Check sheet for the modelled part. Datum: model origin and axes. Units: mm. Face numbers are marked on the shaded views. Round coordinates to 2 decimals unless told otherwise and drop trailing zeros. Order: outer loops, then holes, each group sorted by start corner. A loop starts at its lowest first (then second) coordinate and runs counter-clockwise, first axis right, second up.
Q1. Cross-section at D-D on y = 11. Give the number of separate pieces and of enclosed holes in the cut face, then the cut area to 3 significant figures.
Q2. Cross-section at A-A on x = -100. Record the cut outline in (y, z).
Q3. Cross-section at B-B on z = 20.5. Record the cut outline in (x, y).
Q4. Depth check by flat-ended pin: P1, Ø1.8, axis at x = 0, z = 10, coming from the -Y side; P2, Ø5.5, axis at x = 0, z = -44, coming from the +Y side; P3, Ø3, axis at x = -90.5, y = 10, coming from the -Z side; P4, Ø5, axis at y = 2.5, z = -14.5, coming from the +X side. Enter the tip coordinate at first touch or a pass-through.
Q5. Scan lines: probe 1 along Z at (x, y) = (-70, 9.25); probe 2 along Z at (x, y) = (-70.5, 11.75); probe 3 along X at (y, z) = (7.25, -6). Record each from-to range of solid material in increasing order.
Q6. Cross-section at C-C on x = -53.5. Record the cut outline in (y, z).
Q7. Mould release check, pull along X, two halves, no side actions. Record for the marked faces 1, 2 and 3: +X half, -X half, draft (parallel to the pull), parting line (faces both ways), or undercut.
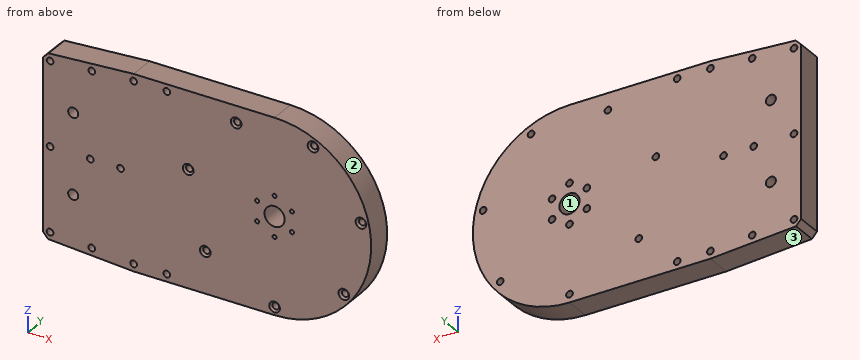
from build123d import *
from OCP.BRepFilletAPI import BRepFilletAPI_MakeChamfer

# Parameters (mm, degrees)
SKETCH1_R                 = 5
SKETCH1_R_2               = 1
BOSS_EXTRUDE1_DEPTH       = 12.7
SKETCH3_R                 = 1
CUT_EXTRUDE1_DEPTH        = 6.35
M4X0_7_TAPPED_HOLE1_D     = 3.3
CHAMFER1_SIZE             = 1
M4X0_7_TAPPED_HOLE2_D     = 3.3
M4X0_7_TAPPED_HOLE2_DEPTH = 10.1
M4X0_7_TAPPED_HOLE2_TIP   = 0.991420021
CHAMFER2_SIZE             = 2.5
CHAMFER2_SIZE2            = 2.68451721
SKETCH7_R                 = 0.25
SKETCH7_R_2               = 1
CUT_EXTRUDE2_DEPTH        = 126.26088775
M4X0_7_TAPPED_HOLE3_D     = 3.3
M4X0_7_TAPPED_HOLE3_DEPTH = 15.5
M4X0_7_TAPPED_HOLE3_TIP   = 0.991420021
M6X1_0_TAPPED_HOLE1_D     = 5
M6X1_0_TAPPED_HOLE1_DEPTH = 17
M6X1_0_TAPPED_HOLE1_TIP   = 1.502151548


with BuildPart() as part:
    # Sketch1 → Boss-Extrude1 (new body)
    with BuildSketch(Plane(origin=(0, 0, 0), x_dir=(1, 0, 0), z_dir=(0, 1, 0))):
        with BuildLine():
            Line((-115, 45), (-115, -45))
            Line((-115, -45), (-70, -48))
            Line((-70, -48), (0, -48))
            ThreePointArc((0, -48), (48, 0), (0, 48))
            Line((0, 48), (-70, 48))
            Line((-70, 48), (-115, 45))
        make_face()
        with Locations(Location((0, 0, 0), (0, 0, 270))):
            Circle(SKETCH1_R, mode=Mode.SUBTRACT)
        with Locations(Location((0, 10, 0), (0, 0, 270))):
            Circle(SKETCH1_R_2, mode=Mode.SUBTRACT)
        with Locations(Location((8.660254038, 5, 0), (0, 0, 270))):
            Circle(SKETCH1_R_2, mode=Mode.SUBTRACT)
        with Locations(Location((8.660254038, -5, 0), (0, 0, 270))):
            Circle(SKETCH1_R_2, mode=Mode.SUBTRACT)
        with Locations(Location((0, -10, 0), (0, 0, 270))):
            Circle(SKETCH1_R_2, mode=Mode.SUBTRACT)
        with Locations(Location((-8.660254038, -5, 0), (0, 0, 270))):
            Circle(SKETCH1_R_2, mode=Mode.SUBTRACT)
        with Locations(Location((-8.660254038, 5, 0), (0, 0, 270))):
            Circle(SKETCH1_R_2, mode=Mode.SUBTRACT)
    extrude(amount=BOSS_EXTRUDE1_DEPTH)

    # Sketch3 → Cut-Extrude1 (cut)
    with BuildSketch(Plane(origin=(0, 12.7, 0), x_dir=(1, 0, 0), z_dir=(0, 1, 0))):
        with Locations(Location((0, 44, 0), (0, 0, 270))):
            Circle(SKETCH3_R)
        with Locations(Location((34.400585229, 27.433551282, 0), (0, 0, 270))):
            Circle(SKETCH3_R)
        with Locations(Location((42.896828136, -9.790921094, 0), (0, 0, 270))):
            Circle(SKETCH3_R)
        with Locations(Location((19.090884521, -39.642630188, 0), (0, 0, 270))):
            Circle(SKETCH3_R)
        with Locations(Location((-19.090884521, -39.642630188, 0), (0, 0, 270))):
            Circle(SKETCH3_R)
        with Locations(Location((-42.896828136, -9.790921094, 0), (0, 0, 270))):
            Circle(SKETCH3_R)
        with Locations(Location((-34.400585229, 27.433551282, 0), (0, 0, 270))):
            Circle(SKETCH3_R)
    extrude(amount=-CUT_EXTRUDE1_DEPTH, mode=Mode.SUBTRACT)

    # M4x0.7 Tapped Hole1 (through all)
    with Locations(Plane(origin=(-19.090884521, 12.7, 39.642630188), x_dir=(0, 0, 1), z_dir=(0, 1, 0))):
        with Locations((0, 0), (-29.851709094, -23.805943615), (-83.642630188, 19.090884521), (-67.07618147, 53.49146975), (-29.851709094, 61.987712657), (0, 38.181769042), (-67.07618147, -15.309700708)):
            Hole(M4X0_7_TAPPED_HOLE1_D / 2)

    # Chamfer1
    chamfer1_edges = [part.edges().sort_by_distance(p)[0] for p in [
        (34.400585229, 0, -25.783551282),
        (0, 0, -42.35),
        (-42.896828136, 0, 11.440921094),
        (-19.090884521, 0, 41.292630188),
        (-34.400585229, 0, -25.783551282),
        (19.090884521, 0, 41.292630188),
        (42.896828136, 0, 11.440921094),
    ]]
    chamfer(chamfer1_edges, length=CHAMFER1_SIZE)

    # M4x0.7 Tapped Hole2
    with Locations(Plane(origin=(0, 12.7, -10), x_dir=(0, 0, 1), z_dir=(0, 1, 0))):
        with Locations((0, 0), (5, -8.660254038), (15, -8.660254038), (20, 0), (15, 8.660254038), (5, 8.660254038)):
            Hole(M4X0_7_TAPPED_HOLE2_D / 2, depth=M4X0_7_TAPPED_HOLE2_DEPTH)
            with Locations((0, 0, -(M4X0_7_TAPPED_HOLE2_DEPTH + M4X0_7_TAPPED_HOLE2_TIP / 2))):  # 118° drill point
                Cone(0, M4X0_7_TAPPED_HOLE2_D / 2, M4X0_7_TAPPED_HOLE2_TIP, mode=Mode.SUBTRACT)

    # Chamfer2: one chamfer whose edges measure the first distance from different faces: ONE call of the kernel's chamfer builder (chamfer() names one face for all edges)
    chamfer2_edges_1 = [part.edges().sort_by_distance(p)[0] for p in [
        (-115, 6.35, 45),
    ]]
    chamfer2_side_1 = [part.faces().sort_by_distance(p)[0] for p in [
        (-115, 6.35, 0),
    ]]
    chamfer2_edges_2 = [part.edges().sort_by_distance(p)[0] for p in [
        (-115, 6.35, -45),
    ]]
    chamfer2_side_2 = [part.faces().sort_by_distance(p)[0] for p in [
        (-92.5, 6.35, -46.5),
    ]]
    chamfer2 = BRepFilletAPI_MakeChamfer(part.part.solid().wrapped)
    for e in chamfer2_edges_1:
        chamfer2.Add(CHAMFER2_SIZE, CHAMFER2_SIZE2, e.wrapped, chamfer2_side_1[0].wrapped)  # the first distance lies on this face
    for e in chamfer2_edges_2:
        chamfer2.Add(CHAMFER2_SIZE, CHAMFER2_SIZE2, e.wrapped, chamfer2_side_2[0].wrapped)  # the first distance lies on this face
    add(Compound.cast(chamfer2.Shape()), mode=Mode.REPLACE)

    # Sketch7 → Cut-Extrude2 (cut, through all)
    with BuildSketch(Plane.XZ):
        with Locations(Location((-111.5, 41.678571429, 0), (0, 0, 270))):
            Circle(SKETCH7_R)
        with Locations(Location((-70, 44.5, 0), (0, 0, 270))):
            Circle(SKETCH7_R)
        with Locations(Location((-53.5, 44.5, 0), (0, 0, 270))):
            Circle(SKETCH7_R)
        with Locations(Location((-90.75, 43.089285714, 0), (0, 0, 270))):
            Circle(SKETCH7_R)
        with Locations(Location((-90.75, -42.904768504, 0), (0, 0, 90))):
            Circle(SKETCH7_R)
        with Locations(Location((-53.5, -44.31548279, 0), (0, 0, 90))):
            Circle(SKETCH7_R)
        with Locations(Location((-70, -44.31548279, 0), (0, 0, 90))):
            Circle(SKETCH7_R)
        with Locations(Location((-111.5, -41.494054218, 0), (0, 0, 90))):
            Circle(SKETCH7_R)
        with Locations(Location((-111.5, 0.092258605, 0), (0, 0, 270))):
            Circle(SKETCH7_R)
        with Locations(Location((-91.5, 0.092258605, 0), (0, 0, 270))):
            Circle(SKETCH7_R)
        with Locations(Location((-76.5, 0.092258605, 0), (0, 0, 270))):
            Circle(SKETCH7_R)
        with Locations(Location((-100, -19.81548279, 0), (0, 0, 270))):
            Circle(SKETCH7_R_2)
        with Locations(Location((-100, 20, 0), (0, 0, 270))):
            Circle(SKETCH7_R_2)
    extrude(amount=-CUT_EXTRUDE2_DEPTH, mode=Mode.SUBTRACT)

    # M4x0.7 Tapped Hole3
    with Locations(Plane(origin=(-90.75, 0, 43.089285714), x_dir=(0, 0, -1), z_dir=(0, -1, 0))):
        with Locations((0, 0), (1.410714285, -20.75), (-1.410714286, 20.75), (-1.410714286, 37.25), (42.997027109, -20.75), (42.997027109, -0.75), (42.997027109, 14.25), (84.583339932, -20.75), (85.994054218, 0), (87.404768504, 20.75), (87.404768504, 37.25)):
            Hole(M4X0_7_TAPPED_HOLE3_D / 2, depth=M4X0_7_TAPPED_HOLE3_DEPTH)
            with Locations((0, 0, -(M4X0_7_TAPPED_HOLE3_DEPTH + M4X0_7_TAPPED_HOLE3_TIP / 2))):  # 118° drill point
                Cone(0, M4X0_7_TAPPED_HOLE3_D / 2, M4X0_7_TAPPED_HOLE3_TIP, mode=Mode.SUBTRACT)

    # M6x1.0 Tapped Hole1
    with Locations(Plane(origin=(-100, 0, 20), x_dir=(0, 0, -1), z_dir=(0, -1, 0))):
        with Locations((0, 0), (39.81548279, 0)):
            Hole(M6X1_0_TAPPED_HOLE1_D / 2, depth=M6X1_0_TAPPED_HOLE1_DEPTH)
            with Locations((0, 0, -(M6X1_0_TAPPED_HOLE1_DEPTH + M6X1_0_TAPPED_HOLE1_TIP / 2))):  # 118° drill point
                Cone(0, M6X1_0_TAPPED_HOLE1_D / 2, M6X1_0_TAPPED_HOLE1_TIP, mode=Mode.SUBTRACT)


solid = part.part
Results found:
1. separate pieces: 1
1. enclosed holes: 27
1. area: 14,200 mm2
2. outline: (0, -46) - (12.7, -46) - (12.7, -22.32) - (0, -22.32) - close; (0, -17.32) - (12.7, -17.32) - (12.7, 17.5) - (0, 17.5) - close; (0, 22.5) - (12.7, 22.5) - (12.7, 46) - (0, 46) - close
3. outline: (-115, 0) - (-102.45, 0) - (-102.45, 12.7) - (-115, 12.7) - close; (-97.55, 0) - (43.4, 0) - (43.4, 12.7) - (-97.55, 12.7) - close
4. P1: passes through
4. P2: stops at y = 12.7
4. P3: stops at z = -46.73
4. P4: stops at x = 46.48
5. probe 1: z = -48 to -45.97, -42.67 to 42.85, 46.15 to 48
5. probe 2: z = -47.97 to -45.89, -42.74 to 42.93, 46.07 to 47.97
5. probe 3: x = -115 to -9.97, -7.35 to 7.35, 9.97 to 47.62
6. outline: (0, -48) - (12.7, -48) - (12.7, -45.97) - (0, -45.97) - close; (0, -42.67) - (12.7, -42.67) - (12.7, 42.85) - (0, 42.85) - close; (0, 46.15) - (12.7, 46.15) - (12.7, 48) - (0, 48) - close
7. face 1: undercut
7. face 2: +X half
7. face 3: -X half
